from build123d import *

# Parameters (mm, degrees)
SKETCH1_R           = 2
BOSS_EXTRUDE1_DEPTH = 2
SKETCH2_R           = 2.391473365
SKETCH2_R_2         = 2
SKETCH2_R_3         = 0.308853545
BOSS_EXTRUDE2_DEPTH = 1
FILLET1_R           = 0.2
SKETCH3_R           = 0.25
BOSS_EXTRUDE3_DEPTH = 2


with BuildPart() as part:
    # Sketch1 → Boss-Extrude1 (new body)
    with BuildSketch(Plane.XY):
        Polygon((0, -7), (5.5, -7), (5.5, 2.5), (2.5, 5.5), (-2.5, 5.5), (-5.5, 2.5), (-5.5, -7), align=None)
        Circle(SKETCH1_R, mode=Mode.SUBTRACT)
    extrude(amount=BOSS_EXTRUDE1_DEPTH)

    # Sketch2 → Boss-Extrude2 (add)
    # profile 1 of 3: a face of its own
    with BuildSketch(Plane.XY.offset(2)):
        Circle(SKETCH2_R)
        Circle(SKETCH2_R_2, mode=Mode.SUBTRACT)
    # profile 2 of 3: a face of its own
    with BuildSketch(Plane.XY.offset(2)):
        with Locations((-4.567781371, -6.437447931)):
            Circle(SKETCH2_R_3)
    # profile 3 of 3: a face of its own
    with BuildSketch(Plane.XY.offset(2)):
        with Locations(Location((4.567781371, -6.437447931, 0), (0, 0, 180))):
            Circle(SKETCH2_R_3)
    extrude(amount=BOSS_EXTRUDE2_DEPTH)

    # Fillet1
    fillet1_edges = [part.edges().sort_by_distance(p)[0] for p in [
        (-2.391473365, 0, 2),
        (-4.876634915, -6.437447931, 2),
        (4.876634915, -6.437447931, 2),
    ]]
    fillet(fillet1_edges, radius=FILLET1_R)

    # Sketch3 → Boss-Extrude3 (add)
    with BuildSketch(Plane.XZ.offset(7)):
        with Locations(Location((0, 1.75, 0), (0, 0, 90))):
            Circle(SKETCH3_R)
        with Locations(Location((2, 1.75, 0), (0, 0, 90))):
            Circle(SKETCH3_R)
        with Locations(Location((-2, 1.75, 0), (0, 0, 180))):
            Circle(SKETCH3_R)
    extrude(amount=BOSS_EXTRUDE3_DEPTH)


solid = part.part
Verification items for the finished model (mm, model axes). A direction names the side the tool comes from. Coordinates: 2 decimals unless noted, no trailing zeros. Order: outer loops, then holes, each group sorted by start corner. A loop starts at its lowest first (then second) coordinate and runs counter-clockwise, first axis right, second up.
Item 1: Access from +Z, -Z, +X, -X, +Y, -Y to the whole of each face (thin tool, end or side, straight path). Record for faces 1 (the face through (0, -3, 2)), 2 (the face through (-1, -2, 0)).
Filled in:
face 1: +Z
face 2: -Z, +X, -X, +Y, -Y
Item 2: Section check B-B, the plane z = 1.75. Enter the section's corners in (x, y), then the cut area to 3 significant figures.
Filled in:
outline: (-5.5, -7) - (-2.25, -7) - (-2.25, -9) - (-1.75, -9) - (-1.75, -7) - (-0.25, -7) - (-0.25, -9) - (0.25, -9) - (0.25, -7) - (1.75, -7) - (1.75, -9) - (2.25, -9) - (2.25, -7) - (5.5, -7) - (5.5, 2.5) - (2.5, 5.5) - (-2.5, 5.5) - (-5.5, 2.5) - close; hole circle Ø4 at (0, 0)
area: 119 mm2
Item 3: Section check A-A, the plane y = 0. Enter the section's corners in (x, z), then the cut area to 3 significant figures.
Filled in:
outline: (-5.5, 0) - (-2, 0) - (-2, 3) - (-2.39, 3) - (-2.39, 2.2) arc R0.2 cw to (-2.59, 2) - (-5.5, 2) - close; (2, 0) - (5.5, 0) - (5.5, 2) - (2.59, 2) arc R0.2 cw to (2.39, 2.2) - (2.39, 3) - (2, 3) - close
area: 14.8 mm2
Item 4: Depth check by flat-ended pin: pin 1 (1.6 mm diameter, centred on x = 1.5, z = 0.5, fed in from -Y); pin 2 (2.5 mm diameter, centred on x = 0, y = 0, fed in from -Z). Enter the tip coordinate at first touch or a pass-through.
Filled in:
pin 1: stops at y = -7
pin 2: passes through
Item 5: Release check for a two-part mould opening along X. For faces 3 (the face through (0, -2, 1)), 4 (the face through (5.5, -2, 1)), 5 (the face through (-5.5, -2, 1)), 6 (the face through (-0.518, -2.335, 2.594)) record: +X half, -X half, draft (parallel to the pull), parting line (faces both ways), or undercut.
Filled in:
face 3: undercut
face 4: +X half
face 5: -X half
face 6: parting line
Item 6: Section check C-C, the plane y = -8. Enter the section's corners in (x, z).
Filled in:
outline: circle Ø0.5 at (-2, 1.75); circle Ø0.5 at (0, 1.75); circle Ø0.5 at (2, 1.75)
Item 7: Section check D-D, the plane z = 0.85. Enter the section's corners in (x, y), then the cut area to 3 significant figures.
Filled in:
outline: (-5.5, -7) - (5.5, -7) - (5.5, 2.5) - (2.5, 5.5) - (-2.5, 5.5) - (-5.5, 2.5) - close; hole circle Ø4 at (0, 0)
area: 116 mm2
Item 8: Material ranges on L1, parallel to Y at x = 0, z = 2.2; L2, parallel to Y at x = 0, z = 1.8; L3, parallel to Z at x = 1, y = -3.75, recorded low to high.
Filled in:
L1: y = -2.39 to -2, 2 to 2.39
L2: y = -9 to -2, 2 to 5.5
L3: z = 0 to 2
